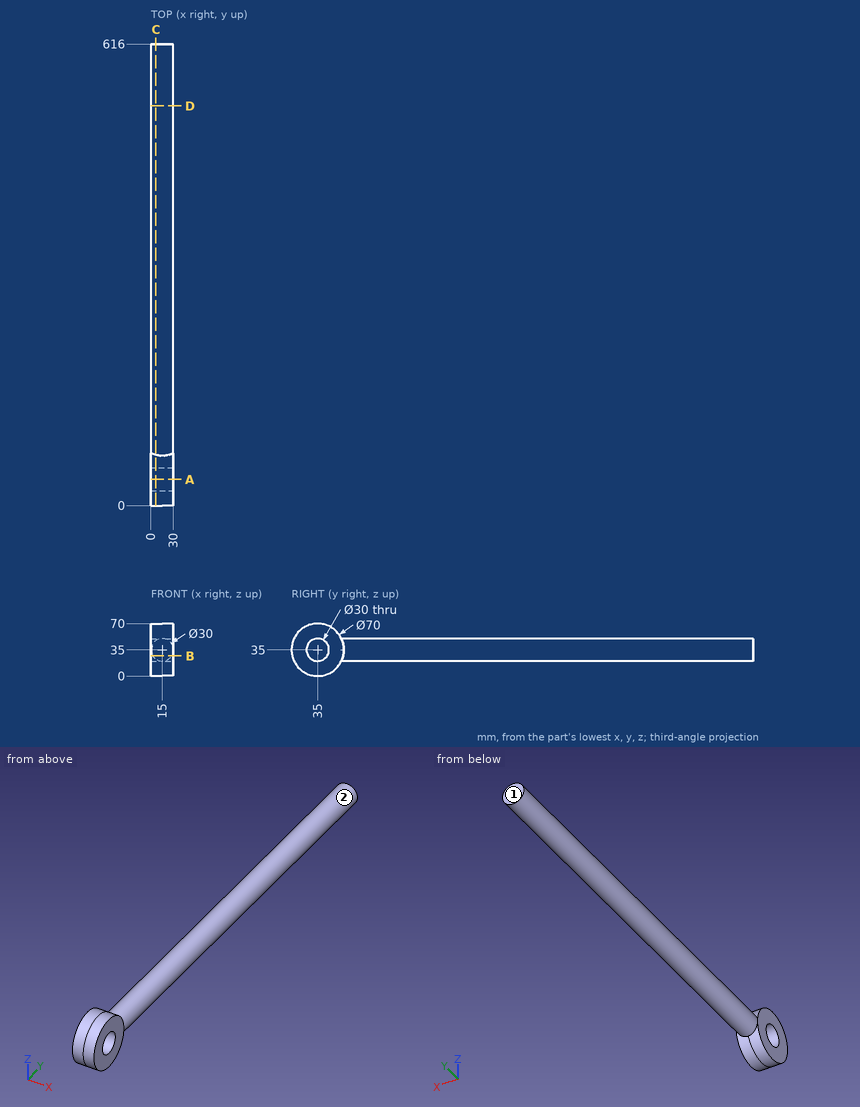
For this review, use the dimensioned drawing (mm, ordinates from the lowest corner) and the shaded views. A direction names the side the tool comes from. Give positions to 0.01 mm unless a question says otherwise; leave off trailing zeros. Order: outer loops, then holes, each group sorted by start corner. A loop starts at its lowest first (then second) coordinate and runs counter-clockwise, first axis right, second up. Notation, with made-up numbers: (86.5, 38) - (93.5, 38) arc R21 ccw to (93.5, 69) - close; hole circle Ø6 at (-14.75, 84.5). An arc over 180 degrees is marked (long way). Use a Markdown table: item, result. Add a question column.
(1) Add section D-D on y = 533.5. Give the boundary of the cut face in (x, z), then the cut area to 3 significant figures.
(2) Machinability: for the marked faces 1 and 2, which of the approach directions +Z, -Z, +X, -X, +Y, -Y give a long, thin tool a straight path to every point of the face, cutting with its end or side? Answer none if there is none.
(3) Add section A-A on y = 35. Give the boundary of the cut face in (x, z).
(4) Wall thickness on probe 1 along Z at (x, y) = (17.5, 35); probe 2 along Z at (x, y) = (14, 392); probe 3 along Y at (x, z) = (25, 41): over which ranges is each line inside the solid? List them lowest first. Write a range as [from, to].
(5) Add section C-C on x = 6.5. Give the boundary of the cut face in (y, z).
(6) Add section B-B on z = 27. Give the boundary of the cut face in (x, y), then the cut area to 3 significant figures.
(7) Clearance check with flat-ended pins moving along their axes: P1, Ø4, axis at x = 26, y = 293.5, coming from the -Z side; P2, Ø1.5, axis at x = 25, y = 283.5, coming from the +Z side; P3, Ø4, axis at x = 11, y = 448, coming from the -Z side. State where each tip first meets the part, or that it passes through.
Report:
| question | item | result |
|---|---|---|
| 1 | outline | circle Ø30 at (15, 35) |
| 1 | area | 707 mm² |
| 2 | face 1 | +Z, -Z, +X, -X, +Y |
| 2 | face 2 | +Y |
| 3 | outline | (0, 0) - (30, 0) - (30, 20) - (0, 20) - close; (0, 50) - (30, 50) - (30, 70) - (0, 70) - close |
| 4 | probe 1 | z = [0, 20], [50, 70] |
| 4 | probe 2 | z = [20.03, 49.97] |
| 4 | probe 3 | y = [0.52, 21.25], [48.75, 616] |
| 5 | outline | (67.75, 22.64) - (616, 22.64) - (616, 47.36) - (67.75, 47.36) arc R35 ccw (long way) to start; hole circle Ø30 at (35, 35) |
| 6 | outline | (0, 0.93) - (30, 0.93) - (30, 22.31) - (0, 22.31) - close; (0, 47.69) - (30, 47.69) - (30, 69.07) - (27.69, 69.07) - (27.69, 616) - (2.31, 616) - (2.31, 69.07) - (0, 69.07) - close |
| 6 | area | 15,200 mm² |
| 7 | P1 | stops at z = 23 |
| 7 | P2 | stops at z = 46.81 |
| 7 | P3 | stops at z = 20.13 |
